```python
from build123d import *

# Parameters (mm, degrees)
BOSS_EXTRUDE1_START = 12.827
BOSS_EXTRUDE1_DEPTH = 3.175
FILLET1_R           = 3.175


with BuildPart() as part:
    # Sketch1 → Boss-Extrude1 (new body)
    with BuildSketch(Plane(origin=(0, 144.904574554, 0), x_dir=(-1, 0, 0), z_dir=(0, -1, 0)).offset(BOSS_EXTRUDE1_START)):
        with BuildLine():
            Line((-107.823062484, -1103.050334154), (0, -1103.050334154))
            Line((0, -1103.050334154), (0, -1338.000334154))
            Line((0, -1338.000334154), (-107.823062484, -1338.000334154))
            Line((-107.823062484, -1338.000334154), (-107.823062484, -1371.337834154))
            ThreePointArc((-107.823062484, -1371.337834154), (-117.348062484, -1380.862834154), (-126.873062484, -1371.337834154))
            Line((-126.873062484, -1371.337834154), (-126.873062484, -1069.712834154))
            ThreePointArc((-126.873062484, -1069.712834154), (-117.348062484, -1060.187834154), (-107.823062484, -1069.712834154))
            Line((-107.823062484, -1069.712834154), (-107.823062484, -1103.050334154))
        make_face()
    extrude(amount=BOSS_EXTRUDE1_DEPTH)

    # Mirror1: part across plane


with BuildPart() as part_1:
    add(part.part)
    add(part.part.mirror(Plane(origin=(0, 0, 0), x_dir=(0, 0, 1), z_dir=(1, 0, 0))))

    # Fillet1
    fillet1_edges = [part_1.edges().sort_by_distance(p)[0] for p in [
        (107.823062484, 130.490074554, 1103.050334154),
        (107.823062484, 130.490074554, 1338.000334154),
        (-107.823062484, 130.490074554, 1338.000334154),
        (-107.823062484, 130.490074554, 1103.050334154),
    ]]
    fillet(fillet1_edges, radius=FILLET1_R)


solid = part_1.part
```
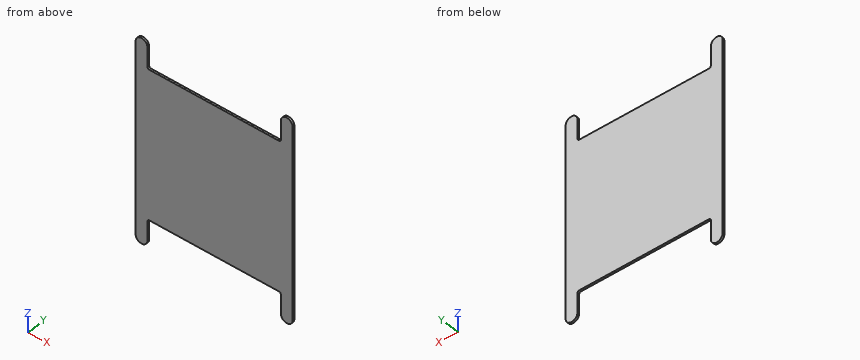
The listing builds one solid part. Answer for the finished solid, in the listing's coordinates (mm). Give positions to 0.01 mm unless a question says otherwise; leave off trailing zeros. Order: outer loops, then holes, each group sorted by start corner. A loop starts at its lowest first (then second) coordinate and runs counter-clockwise, first axis right, second up. Notation, with made-up numbers: (23, 72.25) -> (51, 72.25) arc R22 cw to (51, 106.25) -> close; hole circle Ø11 at (85.5, 47.25). An arc over 180 degrees is marked (long way). One line per item, written item: value.
1) Find section B-B, the plane x = 79. Determine the outline of the cut face in (y, z).
Reported:
outline: (128.9, 1103.05) -> (132.08, 1103.05) -> (132.08, 1338) -> (128.9, 1338) -> close
2) Find section A-A, the plane y = 130.1. Determine the outline of the cut face in (x, z) (3 decimals).
Reported:
outline: (-126.873, 1069.713) arc R9.525 ccw to (-107.823, 1069.713) -> (-107.823, 1099.875) arc R3.175 cw to (-104.648, 1103.05) -> (104.648, 1103.05) arc R3.175 cw to (107.823, 1099.875) -> (107.823, 1069.713) arc R9.525 ccw to (126.873, 1069.713) -> (126.873, 1371.338) arc R9.525 ccw to (107.823, 1371.338) -> (107.823, 1341.175) arc R3.175 cw to (104.648, 1338) -> (-104.648, 1338) arc R3.175 cw to (-107.823, 1341.175) -> (-107.823, 1371.338) arc R9.525 ccw to (-126.873, 1371.338) -> close
3) A flat-ended cylindrical pin translates along its axis: P1, Ø1.5, axis at x = 96, y = 129.5, coming from the +Z side. Find the tip coordinate at first contact, or state that the pin passes through.
Reported:
P1: stops at z = 1338
4) Find the intervals of material crossed by line 1 (X direction, y = 131.75, z = 1090); line 2 (Z direction, x = -38, y = 130.35), in increasing order.
Reported:
line 1: x = -126.87 to -107.82, 107.82 to 126.87
line 2: z = 1103.05 to 1338
